Read the model definition and answer for the solid it produces. Units are mm, in the model's axes. Face numbers are marked on the shaded views. A direction names the side the tool comes from. Give positions to 0.01 mm unless a question says otherwise; leave off trailing zeros. Order: outer loops, then holes, each group sorted by start corner. A loop starts at its lowest first (then second) coordinate and runs counter-clockwise, first axis right, second up. Notation, with made-up numbers: (55, -39.5) - (87, -39.5) arc R9 ccw to (87, -29.5) - close; hole circle Ø3 at (-4.75, 87). An arc over 180 degrees is marked (long way). Write item = value, one per line.
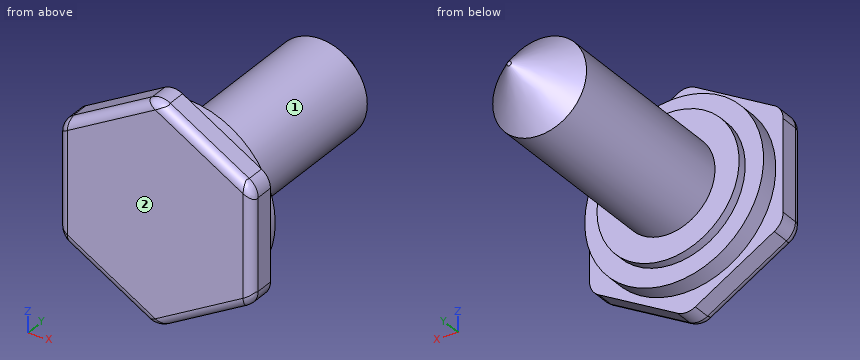
```python
from build123d import *

# Parameters (mm, degrees)
PAD001_DEPTH = 6
SKETCH003_R  = 20
PAD002_DEPTH = 4
SKETCH004_R  = 15.9
PAD003_DEPTH = 2
SKETCH005_R  = 10.5
PAD004_DEPTH = 15
SKETCH006_R  = 10.5
PAD005_DEPTH = 37
CHAMFER_SIZE = 10
FILLET002_R  = 2
FILLET003_R  = 4


with BuildPart() as part:
    # Sketch002 → Pad001 (new body)
    with BuildSketch(Plane.XZ):
        Polygon((21.650635, -12.5), (21.650635, 12.5), (0, 25), (-21.650635, 12.5), (-21.650635, -12.5), (0, -25), align=None)
    extrude(amount=PAD001_DEPTH)

    # Sketch003 → Pad002 (join)
    with BuildSketch(Plane.XZ):
        Circle(SKETCH003_R)
    extrude(amount=-PAD002_DEPTH)

    # Sketch004 (on Face10 of Pad002) → Pad003 (join)
    with BuildSketch(Plane(origin=(0, 4, 0), x_dir=(1, 0, 0), z_dir=(0, 1, 0))):
        Circle(SKETCH004_R)
    extrude(amount=PAD003_DEPTH)

    # Sketch005 (on Face12 of Pad003) → Pad004 (join)
    with BuildSketch(Plane(origin=(0, 6, 0), x_dir=(1, 0, 0), z_dir=(0, 1, 0))):
        Circle(SKETCH005_R)
    extrude(amount=PAD004_DEPTH)

    # Sketch006 (on Face14 of Pad004) → Pad005 (join)
    with BuildSketch(Plane(origin=(0, 21, 0), x_dir=(1, 0, 0), z_dir=(0, 1, 0))):
        Circle(SKETCH006_R)
    extrude(amount=PAD005_DEPTH)

    # Chamfer
    chamfer_edges = [part.edges().sort_by_distance(p)[0] for p in [
        (-10.5, 58, 0),
    ]]
    chamfer(chamfer_edges, length=CHAMFER_SIZE)

    # Fillet002
    fillet002_edges = [part.edges().sort_by_distance(p)[0] for p in [
        (-10.825318, -6, -18.75),
        (-21.650635, -6, 0),
        (-10.825318, -6, 18.75),
        (10.825318, -6, 18.75),
        (21.650635, -6, 0),
        (10.825318, -6, -18.75),
    ]]
    fillet(fillet002_edges, radius=FILLET002_R)

    # Fillet003
    fillet003_edges = [part.edges().sort_by_distance(p)[0] for p in [
        (0, -2, -25),
        (21.650635, -2, -12.5),
        (21.650635, -2, 12.5),
        (-21.650635, -2, -12.5),
        (-21.650635, -2, 12.5),
        (0, -2, 25),
    ]]
    fillet(fillet003_edges, radius=FILLET003_R)


solid = part.part
```
1. Flat-ended cylindrical pins translate along their axes: pin 1 (12 mm diameter, centred on x = 2.5, z = -4.5, fed in from +Y); pin 2 (9.5 mm diameter, centred on x = -7.5, z = 2.5, fed in from +Y); pin 3 (4 mm diameter, centred on x = -3.5, y = 29, fed in from +Z); pin 4 (12 mm diameter, centred on x = -12.5, z = -17, fed in from +Y). Find the tip coordinate at first contact, or state that the pin passes through.
Recorded:
pin_1 = 58
pin_2 = 55.34
pin_3 = 10.39
pin_4 = 6
2. Straight lines are drawn through the part: L1, parallel to Y at x = 15, z = -2; L2, parallel to Y at x = 16, z = 13.5; L3, parallel to Z at x = -7, y = 16. For each, find the intervals that lie inside material, in ascending order. Write a range as [from, to].
Recorded:
L1 = [-6, 6]
L2 = [-6, 0]
L3 = [-7.83, 7.83]
3. Section A-A (y = 32.5) is taken. Determine the outline of the cut face in (x, z), and give its area (3 significant figures).
Recorded:
outline = circle Ø21 at (0, 0)
area = 346 mm^2
4. For the marked faces 1 and 2, determine the directions among +Z, -Z, +X, -X, +Y, -Y from which every point of the face is accessible in a straight line to the end or side of a thin tool.
Recorded:
face_1 = +Y
face_2 = +Z, -Z, +X, -X, -Y
